Input: part model. Units: mm. Frame: model coordinates. Coordinates: 2 decimals unless noted, no trailing zeros. Write each loop counter-clockwise with the first axis right and the second up, starting at its lowest first coordinate (ties: lowest second). Pieces come first, ordered by that corner, then holes. Notation, with made-up numbers: (41.5, -14.75) - (46.5, -14.75) arc R17 ccw to (46.5, 1.25) - close; hole circle Ø9 at (0.5, 13). An arc over 180 degrees is marked (long way). One line per question, with ' | ' between items. Start each with the question number.
1) Section query B-B on x = 12. Return loops of the section in (y, z), and give its area (3 significant figures).
2) Section query C-C on y = 0.85. Give the number of separate pieces and of enclosed holes in the cut face, and give its area (3 significant figures).
3) Section query D-D on z = 20.5. Return loops of the section in (x, y), and give its area (3 significant figures).
4) Section query A-A on z = 76. Return loops of the section in (x, y), and give its area (3 significant figures).
5) First-contact query: P1, Ø1.5, axis at x = 7, y = 2, coming from the +Z side; P2, Ø1.5, axis at y = 1.5, z = 113.5, coming from the -X side. Flat tips, straight axial feed; report the tip coordinate or a pass-through.
6) Line query: line 1 (Z direction, x = 16, y = 2.2); line 2 (Z direction, x = 18.5, y = 0.5); line 3 (Z direction, x = 0, y = 0.6). Output: solid intervals per line, ascending.
Autodesk Inventor part; units mm, degrees
ref_plane "YZ Plane" through (0, 0, 0) normal (1, 0, 0) x (0, 1, 0)
ref_plane "XZ Plane" through (0, 0, 0) normal (0, 1, 0) x (-1, 0, 0)
ref_plane "XY Plane" through (0, 0, 0) normal (0, 0, 1) x (1, 0, 0)
sketch "Sketch1" plane through (0, 0, 0) normal (0, 1, 0) x (-1, 0, 0)
  line L0 (9, 30.5) -> (-9, 30.5) construction
  line L1 (-9, 30.5) -> (-9, -12.5) construction
  line L2 (-9, -30.5) -> (9, -30.5)
  line L3 (9, 30.5) -> (-9, -30.5) construction
  line L4 (-9, 30.5) -> (9, -30.5) construction
  circle A0 centre (0, -24) radius 2
  circle A1 centre (0, 12) radius 2
  line L5 (9, 30.5) -> (-9, 30.5) construction
  line L6 (-33.8261, 11.5) -> (-15.8261, 11.5) construction
  line L7 (-33.8261, 11.5) -> (-9, 54.5)
  line L8 (-15.8261, 11.5) -> (14.1464, 63.4139) construction
  line L9 (-9, 54.5) -> (-33.8261, 97.5)
  line L10 (9, 54.5) -> (-15.8261, 97.5)
  line L11 (-33.8261, 97.5) -> (-15.8261, 97.5)
  line L12 (-15.8261, 11.5) -> (9, 11.5) construction
  line L13 (-9, -12.5) -> (-33.8261, 11.5)
  line L14 (-9, -12.5) -> (-9, -30.5)
  line L15 (9, -30.5) -> (9, 11.5)
  line L16 (9, 11.5) -> (9, 54.5)
  point P0 (0, 0)
  dimension "d0" = 18
  dimension "d1" = 61
  dimension "d2" = 4
  dimension "d3" = 24
  dimension "d4" = 4
  dimension "d5" = 36
  dimension "d8" = 18
  dimension "d9" = 43
  dimension "d10" = 60
  dimension "d11" = 120
  dimension "d14" = 18
  dimension "d15" = 24
extrude "Extrusion1" add sketch "Sketch1" along normal blind 3
fillet "Fillet1" radius 16 1 edges at (33.8261, 1.5, 11.5)
fillet "Fillet2" radius 4 1 edges at (9, 1.5, 54.5)
fillet "Fillet3" radius 2 1 edges at (33.8261, 1.5, 97.5)
fillet "Fillet4" radius 4 2 edges at (15.8261, 1.5, 97.5) (-9, 1.5, 54.5)
fillet "Fillet5" radius 9 2 edges at (9, 1.5, -30.5) (-9, 1.5, -30.5)
sketch "Sketch2" plane through (0, 3, 0) normal (0, 1, 0) x (1, 0, 0)
  arc A0 (9, 21.5) -> (-9, 21.5) centre (0, 21.5) ccw construction
  line L0 (-9, 21.5) -> (-9, -53.4282) construction
  arc A1 (-9, -53.4282) -> (-8.4641, -55.4282) centre (-5, -53.4282) ccw construction
  line L1 (-8.4641, -55.4282) -> (14.6714, -95.5) construction
  arc A2 (14.6714, -95.5) -> (18.1355, -97.5) centre (18.1355, -93.5) ccw construction
  line L2 (18.1355, -97.5) -> (30.362, -97.5) construction
  arc A3 (30.362, -97.5) -> (32.094, -94.5) centre (30.362, -95.5) ccw construction
  line L3 (32.094, -94.5) -> (10.1547, -56.5) construction
  arc A4 (10.1547, -52.5) -> (10.1547, -56.5) centre (13.6188, -54.5) ccw construction
  line L4 (10.1547, -52.5) -> (27.5792, -22.3198) construction
  arc A5 (27.5792, -22.3198) -> (24.8435, -2.8164) centre (13.7228, -14.3198) ccw construction
  line L5 (24.8435, -2.8164) -> (9, 12.5) construction
  line L6 (9, 12.5) -> (9, 21.5) construction
  circle A6 centre (0, -12) radius 2 construction
  circle A7 centre (0, 24) radius 2 construction
  line L7 (5.6099, 10.2137) -> (22.0634, -5.6922) construction
  arc A8 (24.1151, -20.3198) -> (22.0634, -5.6922) centre (13.7228, -14.3198) ccw construction
  line L8 (24.1151, -20.3198) -> (6.6906, -50.5) construction
  arc A9 (6.6906, -50.5) -> (6.6906, -58.5) centre (13.6188, -54.5) ccw construction
  line L9 (6.6906, -58.5) -> (26.8979, -93.5) construction
  line L10 (26.8979, -93.5) -> (18.1355, -93.5)
  line L11 (18.1355, -93.5) -> (-5, -53.4282)
  line L12 (-5, -53.4282) -> (-5, 21.5)
  arc A10 (5, 21.5) -> (-5, 21.5) centre (0, 21.5) ccw
  line L13 (5, 21.5) -> (5, 11.6517) construction
  circle A11 centre (5, 10.8034) radius 2
  arc A12 (5, 11.6517) -> (5.6099, 10.2137) centre (7, 11.6517) ccw construction
  circle A13 centre (22.0634, -5.6922) radius 2
  circle A14 centre (17.0829, -32.5) radius 2
  circle A15 centre (6.6906, -50.5) radius 2
  circle A16 centre (26.8979, -93.5) radius 2
  circle A17 centre (16.7942, -76) radius 2
  point P0 (0, 0)
  dimension "d22" = 4
  dimension "d23" = 4
  dimension "d26" = 2
  dimension "d27" = 4
  dimension "d28" = 4
  dimension "d29" = 4
  dimension "d30" = 4
  dimension "d40" = 18
  dimension "d41" = 4
sketch "Sketch3" plane through (0, 3, 0) normal (0, 1, 0) x (1, 0, 0)
  arc A0 (30.362, -97.5) -> (32.094, -94.5) centre (30.362, -95.5) ccw
  line L0 (32.362, -95.5) -> (32.362, -127.5)
  line L1 (32.362, -127.5) -> (14.6714, -127.5)
  arc A1 (14.6714, -95.5) -> (18.1355, -97.5) centre (18.1355, -93.5) ccw
  line L2 (14.6714, -127.5) -> (14.6714, -95.5)
  line L3 (18.1355, -97.5) -> (30.362, -97.5)
  point P0 (0, 0)
  dimension "d31" = 32
extrude "Extrusion3" add sketch "Sketch3" against normal up to surface (3 mm away)
fillet "Fillet6" radius 4 3 edges at (14.6714, 1.5, 95.5) (14.6714, 1.5, 127.5) (32.362, 1.5, 127.5)
extrude "Extrusion2" cut sketch "Sketch2" against normal through all contours A14 | A15 | A17
sketch "Sketch4" plane through (0, 3, 0) normal (0, 1, 0) x (1, 0, 0)
  circle A0 centre (28.362, -123.5) radius 2
  line L0 (32.362, -123.5) -> (32.362, -95.5)
  line L1 (18.6714, -127.5) -> (28.362, -127.5)
  point P0 (0, 0)
  dimension "d35" = 4
  dimension "d36" = 4
  dimension "d37" = 4
extrude "Extrusion4" cut sketch "Sketch4" against normal through all
equation "\"d11\" = 2 * d10"
properties part number "ClawGrabPlate" material "Aluminum 6061"
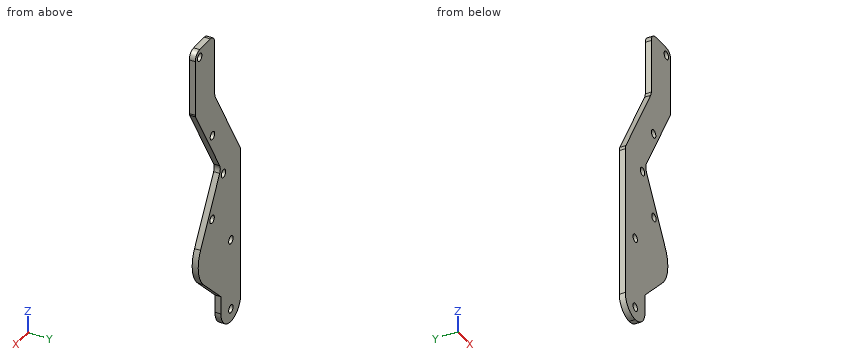
Answer key:
1) outline: (0, -9.6) - (3, -9.6) - (3, 49.3) - (0, 49.3) - close; (0, 59.7) - (3, 59.7) - (3, 90.87) - (0, 90.87) - close | area: 270 mm²
2) separate pieces: 1 | enclosed holes: 6 | area: 3,520 mm²
3) outline: (-9, 0) - (28.48, 0) - (28.48, 3) - (-9, 3) - close | area: 112 mm²
4) outline: (3.41, 0) - (14.79, 0) - (14.79, 3) - (3.41, 3) - close; (18.79, 0) - (21.41, 0) - (21.41, 3) - (18.79, 3) - close | area: 42.0 mm²
5) P1: z = 83.51 | P2: x = 14.67
6) line 1: -5.73 to 30.82, 34.18 to 42.38, 66.62 to 74.16, 77.84 to 126.48 | line 2: -3.32 to 31.09, 33.91 to 38.05, 70.95 to 74.96, 77.04 to 127.5 | line 3: -30.5 to -26, -22 to 10, 14 to 70.09
